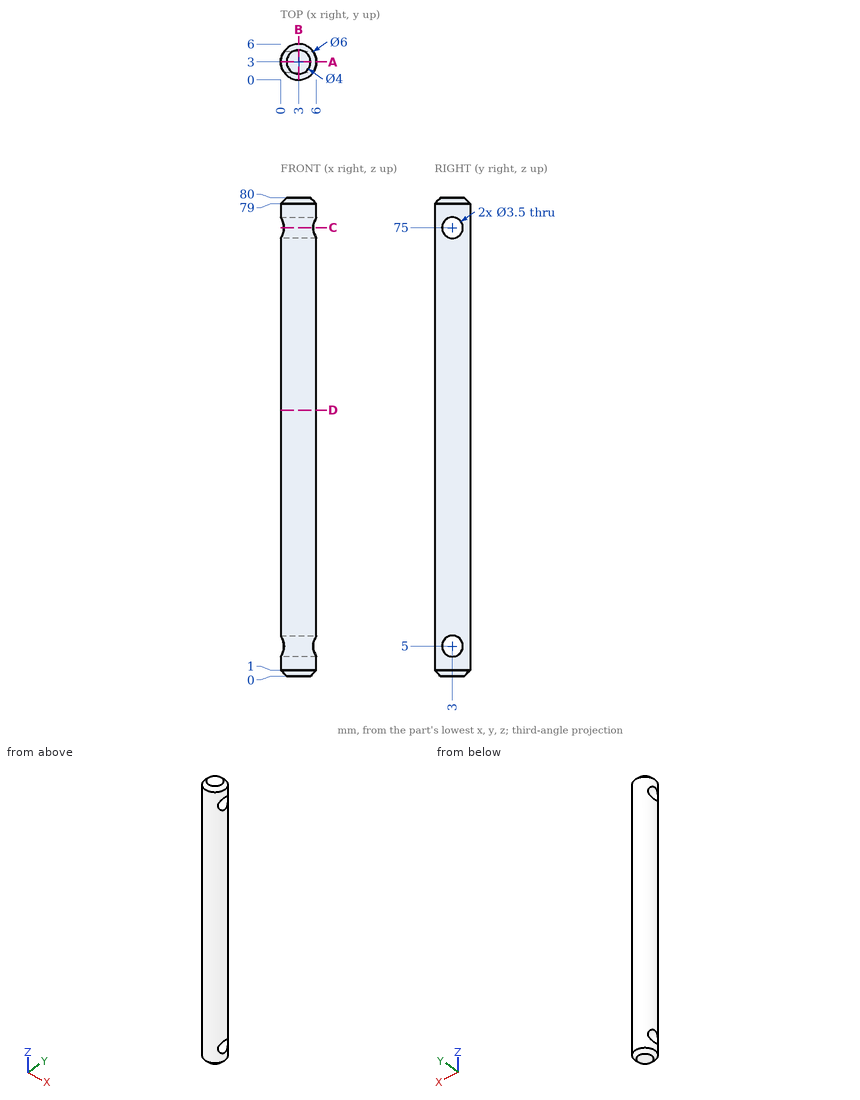
Print and shaded views of the part. All mm, measured from the part's lowest x, y and z. Coordinates: 2 decimals unless noted, no trailing zeros. Order: outer loops, then holes, each group sorted by start corner. A loop starts at its lowest first (then second) coordinate and runs counter-clockwise, first axis right, second up. Notation, with made-up numbers: (22.5, 52.25) - (35.5, 52.25) arc R27 ccw to (35.5, 72.25) - close; hole circle Ø10 at (80.5, 83.25). An arc over 180 degrees is marked (long way). Put each result on its own line as item: value.
1. Saw through at C-C (z = 75). Write the cut outline in (x, y).
Answer sheet:
outline: (0.56, 1.25) arc R3 ccw to (5.44, 1.25) - close; (0.56, 4.75) - (5.44, 4.75) arc R3 ccw to start
2. Probe line 1 along Y through (x, z) = (2.75, 5); line 2 along Z through (x, y) = (4, 1.75); line 3 along Z through (x, y) = (5.5, 4). List the from-to ranges inside material, lowest first. Write a range as [from, to].
Answer sheet:
line 1: y = [0.01, 1.25], [4.75, 5.99]
line 2: z = [0, 3.78], [6.22, 73.78], [76.22, 80]
line 3: z = [0.69, 3.56], [6.44, 73.56], [76.44, 79.31]
3. Saw through at B-B (x = 3). Write the cut outline in (y, z), and give its area (3 significant figures).
Answer sheet:
outline: (0, 1) - (1, 0) - (5, 0) - (6, 1) - (6, 79) - (5, 80) - (1, 80) - (0, 79) - close; hole circle Ø3.5 at (3, 5); hole circle Ø3.5 at (3, 75)
area: 459 mm^2
4. Saw through at A-A (y = 3). Write the cut outline in (x, z).
Answer sheet:
outline: (0, 1) - (1, 0) - (5, 0) - (6, 1) - (6, 3.25) - (0, 3.25) - close; (0, 6.75) - (6, 6.75) - (6, 73.25) - (0, 73.25) - close; (0, 76.75) - (6, 76.75) - (6, 79) - (5, 80) - (1, 80) - (0, 79) - close
5. Saw through at D-D (z = 44.5). Write the cut outline in (x, y), and give its area (3 significant figures).
Answer sheet:
outline: circle Ø6 at (3, 3)
area: 28.3 mm^2
6. Drop flat-ended pins along their axis: P1, Ø3, axis at y = 3, z = 75, coming from the -X side; P2, Ø2, axis at x = 4.5, z = 18, coming from the -Y side. Give the stop position or say it passes through.
Answer sheet:
P1: passes through
P2: stops at y = 0.04
